Check sheet for the modelled part. Datum: model origin and axes. Units: mm. A direction names the side the tool comes from. Round coordinates to 2 decimals unless told otherwise and drop trailing zeros. Loops run counter-clockwise (first coordinate to the right, second up) from the corner with the lowest first, then second, coordinate; pieces in that order, holes last. Notation, with made-up numbers: (39, -9.75) - (83, -9.75) arc R19 ccw to (83, 10.25) - close; hole circle Ø10 at (51, 26). An arc over 180 degrees is marked (long way). Put each result on its own line as item: value. Start each with the question number.
```python
from build123d import *

# Parameters (mm, degrees)
BOSS_EXTRUDE1_DEPTH                            = 23
CSK_FOR_4_FLAT_HEAD_MACHINE_SCREW1_D           = 3.4544
CSK_FOR_4_FLAT_HEAD_MACHINE_SCREW1_DEPTH       = 3.5
CSK_FOR_4_FLAT_HEAD_MACHINE_SCREW1_CSINK_D     = 5.715
CSK_FOR_4_FLAT_HEAD_MACHINE_SCREW1_CSINK_ANGLE = 82
SKETCH5_R                                      = 9.3
BOSS_EXTRUDE2_DEPTH                            = 2
BOSS_EXTRUDE2_DEPTH_BACK                       = 4
BOSS_EXTRUDE3_DEPTH                            = 2
CUT_EXTRUDE1_DEPTH                             = 3.6
SKETCH8_R                                      = 1.725
CUT_EXTRUDE2_DEPTH                             = 9


with BuildPart() as part:
    # Base → Boss-Extrude1 (new body)
    with BuildSketch(Plane.XY):
        with BuildLine():
            Line((-5.31789432, 9.4), (5.31789432, 9.4))
            ThreePointArc((5.31789432, 9.4), (0, -10.8), (-5.31789432, 9.4))
        make_face()
        with BuildLine():
            Line((-5.253570215, 5.9), (5.253570215, 5.9))
            ThreePointArc((5.253570215, 5.9), (0, -7.9), (-5.253570215, 5.9))
        make_face(mode=Mode.SUBTRACT)
    extrude(amount=BOSS_EXTRUDE1_DEPTH)

    # CSK for #4 Flat Head Machine Screw1
    with Locations(Plane(origin=(0, 9.4, 0), x_dir=(1, 0, 0), z_dir=(0, 1, 0))):
        with Locations((0, -11)):
            CounterSinkHole(CSK_FOR_4_FLAT_HEAD_MACHINE_SCREW1_D / 2, CSK_FOR_4_FLAT_HEAD_MACHINE_SCREW1_CSINK_D / 2, depth=CSK_FOR_4_FLAT_HEAD_MACHINE_SCREW1_DEPTH, counter_sink_angle=CSK_FOR_4_FLAT_HEAD_MACHINE_SCREW1_CSINK_ANGLE)

    # Sketch5 → Boss-Extrude2 (add, two sides)
    with BuildSketch(Plane.XY.offset(23)) as boss_extrude2_sk:
        Circle(SKETCH5_R)
    extrude(amount=BOSS_EXTRUDE2_DEPTH)
    extrude(boss_extrude2_sk.sketch, amount=-BOSS_EXTRUDE2_DEPTH_BACK)

    # Sketch6 → Boss-Extrude3 (add)
    with BuildSketch(Plane.XY.offset(25)):
        Polygon((0, 8.544783984), (-7.4, 4.272391992), (-7.4, -4.272391992), (0, -8.544783984), (7.4, -4.272391992), (7.4, 4.272391992), align=None)
    extrude(amount=BOSS_EXTRUDE3_DEPTH)

    # Sketch7 → Cut-Extrude1 (cut)
    with BuildSketch(Plane(origin=(0, 0, 19), x_dir=(-1, 0, 0), z_dir=(0, 0, -1))):
        Polygon((0, 3.868246804), (-3.35, 1.934123402), (-3.35, -1.934123402), (0, -3.868246804), (3.35, -1.934123402), (3.35, 1.934123402), align=None)
    extrude(amount=-CUT_EXTRUDE1_DEPTH, mode=Mode.SUBTRACT)

    # Sketch8 → Cut-Extrude2 (cut, through all)
    with BuildSketch(Plane(origin=(0, 0, 19), x_dir=(-1, 0, 0), z_dir=(0, 0, -1))):
        Circle(SKETCH8_R)
    extrude(amount=-CUT_EXTRUDE2_DEPTH, mode=Mode.SUBTRACT)


solid = part.part
```
Q1. Cross-section at D-D on x = 8.75. Enter the section's corners in (y, z), and give its area (3 significant figures).
Q2. Cross-section at B-B on y = 0. Enter the section's corners in (x, z) (3 decimals).
Q3. Set-up check for faces 1 (the face through (3, -7, 25)), 2 (the face through (-3.75, -6.38, 25.99)), 3 (the face through (3.75, 6.38, 25.99)), 4 (the face through (0.225, 6.984, 9.287)), 5 (the face through (1.698, -2.888, 20.775)): record each of +Z, -Z, +X, -X, +Y, -Y from which the full face is reachable in a straight line by a thin tool's end or side.
Q4. Depth check by flat-ended pin: pin 1 Ø3 at (y, z) = (-2.5, 14) entering from +X; pin 2 Ø1 at (y, z) = (-0.5, 26.5) entering from +X; pin 3 Ø2 at (y, z) = (0.5, 26.5) entering from -X. Enter the tip coordinate at first touch or a pass-through.
Q5. Cross-section at A-A on z = 21.5. Enter the section's corners in (x, y), and give its area (3 significant figures).
Q6. Material ranges on line 1 (X direction, y = 0, z = 4); line 2 (Y direction, x = 0, z = 24.4) (3 decimals); line 3 (Z direction, x = -5, y = 8), recorded low to high. Write a range as from..to.
Q7. Draft check along Y on faces 6 (the face through (0.397, -10.793, 11.339)), 7 (the face through (7.4, 0, 26)), 8 (the face through (3.35, 0, 21)), 9 (the face through (-1, 9.4, 14)). Enter one of: +Y half, -Y half, draft (parallel to the pull), parting line (faces both ways), or undercut.
Q8. Cross-section at C-C on z = 11. Enter the section's corners in (x, y).
Answer list:
1. outline: (-6.33, 0) - (6.33, 0) - (6.33, 23) - (3.15, 23) - (3.15, 25) - (-3.15, 25) - (-3.15, 23) - (-6.33, 23) - close
1. area: 304 mm2
2. outline: (-10.8, 0) - (-7.9, 0) - (-7.9, 19) - (-3.35, 19) - (-3.35, 22.6) - (-1.725, 22.6) - (-1.725, 27) - (-7.4, 27) - (-7.4, 25) - (-9.3, 25) - (-9.3, 23) - (-10.8, 23) - close; (1.725, 22.6) - (3.35, 22.6) - (3.35, 19) - (7.9, 19) - (7.9, 0) - (10.8, 0) - (10.8, 23) - (9.3, 23) - (9.3, 25) - (7.4, 25) - (7.4, 27) - (1.725, 27) - close
3. face 1: +Z
3. face 2: +Z, -X, -Y
3. face 3: +Z, +X, +Y
3. face 4: +Y
3. face 5: -Z
4. pin 1: stops at x = 10.75
4. pin 2: stops at x = 7.4
4. pin 3: stops at x = -7.4
5. outline: (-5.32, 9.4) arc R10.8 ccw (long way) to (5.32, 9.4) - close; hole (-3.35, -1.93) - (0, -3.87) - (3.35, -1.93) - (3.35, 1.93) - (0, 3.87) - (-3.35, 1.93) - close
5. area: 317 mm2
6. line 1: x = -10.8..-7.9, 7.9..10.8
6. line 2: y = -9.3..-1.725, 1.725..9.3
6. line 3: z = 0..23
7. face 6: parting line
7. face 7: draft
7. face 8: undercut
7. face 9: +Y half
8. outline: (-5.32, 9.4) arc R10.8 ccw (long way) to (5.32, 9.4) - (2.86, 9.4) - (1.73, 8.1) - (1.73, 5.9) - (5.25, 5.9) arc R7.9 cw (long way) to (-5.25, 5.9) - (-1.73, 5.9) - (-1.73, 8.1) - (-2.86, 9.4) - close
